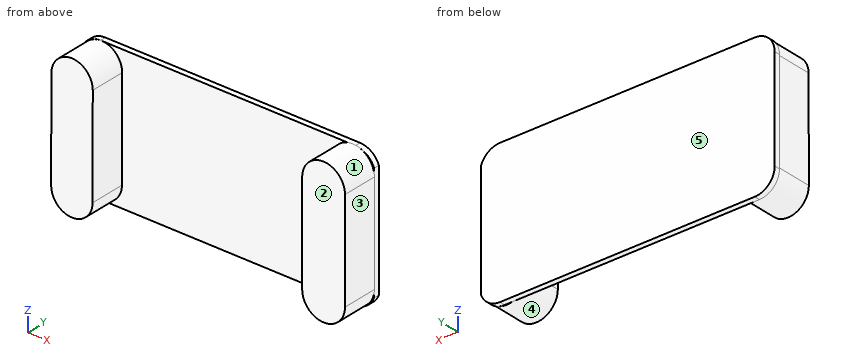
```python
from build123d import *

# Parameters (mm, degrees)
BOSS_EXTRUDE1_DEPTH = 4.5
BOSS_EXTRUDE2_DEPTH = 3.8
BOSS_EXTRUDE3_DEPTH = 12.4
SKETCH5_W           = 103.25
SKETCH5_H           = 49.520314098
BOSS_EXTRUDE4_DEPTH = 2
FILLET1_R           = 7
SKETCH6_W           = 74.836382047
SKETCH6_H           = 26.769621583
CUT_EXTRUDE1_DEPTH  = 0.42
SKETCH7_W           = 32.821875261
SKETCH7_H           = 64.99782183
CUT_EXTRUDE4_DEPTH  = 8.3
BOSS_EXTRUDE5_DEPTH = 12.4


with BuildPart() as part:
    # Sketch1 → Boss-Extrude1 (new body)
    with BuildSketch(Plane(origin=(0, 0, 0), x_dir=(1, 0, 0), z_dir=(0, 1, 0))):
        with BuildLine():
            Line((7.25, 0), (7.25, -35))
            ThreePointArc((7.25, -35), (0, -42.25), (-7.25, -35))
            Line((-7.25, -35), (-7.25, 0))
            ThreePointArc((-7.25, 0), (0, 7.25), (7.25, 0))
        make_face()
    extrude(amount=BOSS_EXTRUDE1_DEPTH)

    # Sketch3 → Boss-Extrude2 (add)
    with BuildSketch(Plane(origin=(0, 4.5, 0), x_dir=(1, 0, 0), z_dir=(0, 1, 0))):
        with BuildLine():
            Line((-2.622571491, -0.457666807), (-2.622571491, -0.011296081))
            Line((-2.622571491, -0.011296081), (2.763792269, -0.011296081))
            Line((2.763792269, -0.011296081), (2.763792269, -0.457666807))
            ThreePointArc((2.763792269, -0.457666807), (2.791332039, -0.235236185), (2.800532634, -0.011296081))
            ThreePointArc((2.800532634, -0.011296081), (-0.153329714, 2.709425568), (-2.622571491, -0.457666807))
        make_face()
        with BuildLine():
            Line((2.763792269, -0.011296081), (-2.622571491, -0.011296081))
            Line((-2.622571491, -0.011296081), (-2.622571491, -0.457666807))
            ThreePointArc((-2.622571491, -0.457666807), (0.070610389, -2.741218326), (2.763792269, -0.457666807))
            Line((2.763792269, -0.457666807), (2.763792269, -0.011296081))
        make_face()
        with BuildLine():
            ThreePointArc((2.763792269, -0.457666807), (0.070610389, -2.741218326), (-2.622571491, -0.457666807))
            Line((-2.622571491, -0.457666807), (-2.622571491, -35.011296081))
            ThreePointArc((-2.622571491, -35.011296081), (0.070610389, -32.318114201), (2.763792269, -35.011296081))
            Line((2.763792269, -35.011296081), (2.763792269, -0.457666807))
        make_face()
        with BuildLine():
            ThreePointArc((2.763792269, -35.011296081), (0.070610389, -32.318114201), (-2.622571491, -35.011296081))
            Line((-2.622571491, -35.011296081), (2.763792269, -35.011296081))
        make_face()
        with BuildLine():
            Line((2.763792269, -35.011296081), (-2.622571491, -35.011296081))
            ThreePointArc((-2.622571491, -35.011296081), (0.070610389, -37.704477961), (2.763792269, -35.011296081))
        make_face()
    extrude(amount=BOSS_EXTRUDE2_DEPTH)

    # Sketch4 → Boss-Extrude3 (add)
    with BuildSketch(Plane(origin=(0, 8.3, 0), x_dir=(1, 0, 0), z_dir=(0, 1, 0))):
        with BuildLine():
            Line((7.25308141, 0.014627933), (7.323691799, -34.996668148))
            ThreePointArc((7.323691799, -34.996668148), (0.085238322, -42.264377491), (-7.182471021, -35.025924014))
            Line((-7.182471021, -35.025924014), (-7.25308141, -0.014627933))
            ThreePointArc((-7.25308141, -0.014627933), (-0.014627933, 7.25308141), (7.25308141, 0.014627933))
        make_face()
    extrude(amount=BOSS_EXTRUDE3_DEPTH)

    # Sketch5 → Boss-Extrude4 (add)
    with BuildSketch(Plane(origin=(0, 20.7, 0), x_dir=(1, 0, 0), z_dir=(0, 1, 0))):
        with Locations((44.371903839, -17.507075639)):
            Rectangle(SKETCH5_W, SKETCH5_H)
    extrude(amount=BOSS_EXTRUDE4_DEPTH)

    # Fillet1
    fillet1_edges = [part.edges().sort_by_distance(p)[0] for p in [
        (95.996903839, 21.7, 42.267232688),
        (95.996903839, 21.7, -7.25308141),
        (-7.253096161, 21.7, -7.25308141),
        (-7.253096161, 21.7, 42.267232688),
    ]]
    fillet(fillet1_edges, radius=FILLET1_R)

    # Sketch6 → Cut-Extrude1 (cut)
    with BuildSketch(Plane(origin=(95.996903839, 0, 0), x_dir=(0, 0, -1), z_dir=(1, 0, 0))):
        with Locations((-22.928368507, 17.221399119)):
            Rectangle(SKETCH6_W, SKETCH6_H)
    extrude(amount=-CUT_EXTRUDE1_DEPTH, mode=Mode.SUBTRACT)

    # Sketch7 → Cut-Extrude4 (cut)
    with BuildSketch(Plane.XZ):
        with Locations((-1.71559597, 16.327002209)):
            Rectangle(SKETCH7_W, SKETCH7_H)
    extrude(amount=-CUT_EXTRUDE4_DEPTH, mode=Mode.SUBTRACT)

    # Sketch9 → Boss-Extrude5 (add)
    with BuildSketch(Plane.XZ.offset(-20.7)):
        with BuildLine():
            Line((80.676554066, 0), (80.676554066, 35.01))
            ThreePointArc((80.676554066, 35.01), (88.176554066, 42.51), (95.676554066, 35.01))
            Line((95.676554066, 35.01), (95.676554066, 0))
            ThreePointArc((95.676554066, 0), (88.176554066, -7.5), (80.676554066, 0))
        make_face()
    extrude(amount=BOSS_EXTRUDE5_DEPTH)


solid = part.part
```
Model file for the job. Use its own axes, mm. Face numbers are marked on the shaded views. A direction names the side the tool comes from. Coordinates: 2 decimals unless noted, no trailing zeros. Loops run counter-clockwise (first coordinate to the right, second up) from the corner with the lowest first, then second, coordinate; pieces in that order, holes last. Notation, with made-up numbers: (26, 59.5) - (68, 59.5) arc R13 ccw to (68, 77.5) - close; hole circle Ø2 at (21, -23.5). An arc over 180 degrees is marked (long way). Write item = value, one per line. Start each with the question number.
Item 1: Drop flat-ended pins along their axis: pin 1 Ø1 at (x, z) = (31, 11.5) entering from -Y; pin 2 Ø2 at (x, y) = (32, 21.5) entering from -Z; pin 3 Ø0.6 at (x, y) = (38.5, 22) entering from +Z. Give the stop position or say it passes through.
Item 2: Pull direction X, two halves, no side cores. Call the marked faces 3, 4 and 5: +X half, -X half, draft (parallel to the pull), parting line (faces both ways), or undercut.
Item 3: 3-axis set-ups, long thin cutter, end or side, ignore diameter. For the marked faces 1 and 2: which of +Z, -Z, +X, -X, +Y, -Y reach the whole face in a straight line?
Item 4: Saw through at C-C, the plane x = 36.5. List the corners of the cut face in (y, z), then the cut area to 3 significant figures.
Item 5: Saw through at A-A, the plane y = 15.5. List the corners of the cut face in (x, z), then the cut area to 3 significant figures.
Item 6: Saw through at B-B, the plane z = 33.5. List the corners of the cut face in (x, y), then the cut area to 3 significant figures.
Item 7: Wall check: probe 1 along X at (y, z) = (10.5, 29.5); probe 2 along X at (y, z) = (18.75, 0.5); probe 3 along Y at (x, z) = (13, 19). Give the ranges that are in metal, low to high. Write a range as [from, to].
Answers:
q1.pin_1 = 20.7
q1.pin_2 = -7.25
q1.pin_3 = 42.27
q2.face_3 = +X half
q2.face_4 = undercut
q2.face_5 = draft
q3.face_1 = +Z, -Y
q3.face_2 = +Z, -Z, +X, -X, -Y
q4.outline = (20.7, -7.25) - (22.7, -7.25) - (22.7, 42.27) - (20.7, 42.27) - close
q4.area = 99.0 mm2
q5.outline = (-7.25, 0.01) arc R7.25 ccw to (7.25, -0.01) - (7.32, 35) arc R7.25 ccw to (-7.18, 35.03) - close; (80.68, 0) arc R7.5 ccw to (95.68, 0) - (95.68, 35.01) arc R7.5 ccw to (80.68, 35.01) - close
q5.area = 1,380 mm2
q6.outline = (-7.25, 20.7) - (-7.19, 20.7) - (-7.19, 8.3) - (7.32, 8.3) - (7.32, 20.7) - (80.68, 20.7) - (80.68, 8.3) - (95.68, 8.3) - (95.68, 20.7) - (95.58, 20.7) - (95.58, 22.7) - (-7.25, 22.7) - close
q6.area = 572 mm2
q7.probe_1 = [-7.19, 7.31], [80.68, 95.68]
q7.probe_2 = [-7.25, 7.25], [80.68, 95.68]
q7.probe_3 = [20.7, 22.7]
